from build123d import *

# Parameters (mm, degrees)
SKETCH_1_R          = 1.5
EXTRUDE_1_DEPTH     = 40
SKETCH_2_R          = 2.75
EXTRUDE_2_DEPTH     = 2.93
CUT_EXTRUDE_1_DEPTH = 1.3


with BuildPart() as part:
    # 草图1 → 凸台-拉伸1 (new body)
    with BuildSketch(Plane(origin=(0, 0, 0), x_dir=(1, 0, 0), z_dir=(0, 1, 0))):
        Circle(SKETCH_1_R)
    extrude(amount=EXTRUDE_1_DEPTH)

    # 草图2 → 凸台-拉伸2 (add)
    with BuildSketch(Plane(origin=(0, 40, 0), x_dir=(1, 0, 0), z_dir=(0, 1, 0))):
        Circle(SKETCH_2_R)
    extrude(amount=EXTRUDE_2_DEPTH)

    # 草图3 → 切除-拉伸1 (cut)
    with BuildSketch(Plane(origin=(0, 42.93, 0), x_dir=(1, 0, 0), z_dir=(0, 1, 0))):
        Polygon((1.024005842, -1.017224346), (1.392945046, 0.378202899), (0.368939204, 1.395427245), (-1.024005842, 1.017224346), (-1.392945046, -0.378202899), (-0.368939204, -1.395427245), align=None)
    extrude(amount=-CUT_EXTRUDE_1_DEPTH, mode=Mode.SUBTRACT)


solid = part.part
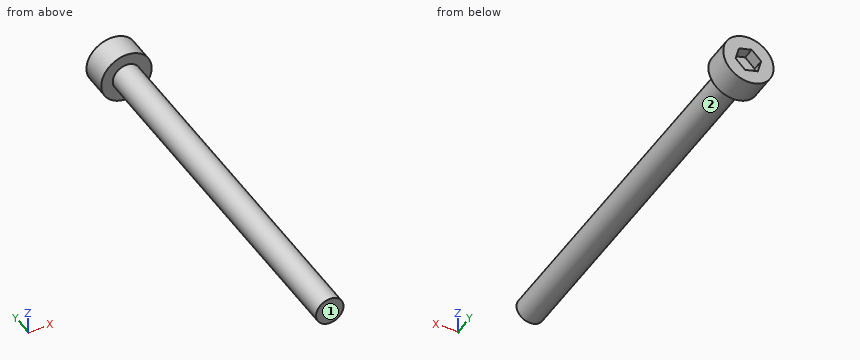
Here's how the part is built. I have some questions about the finished solid (model axes, mm). Face numbers are marked on the shaded views. A direction names the side the tool comes from. Round coordinates to 2 decimals unless told otherwise and drop trailing zeros. Write each loop counter-clockwise with the first axis right and the second up, starting at its lowest first coordinate (ties: lowest second). Pieces come first, ordered by that corner, then holes.
1. Suppose I cut it at A-A (x = 0). List the corners of the cut face in (y, z) for me, and give its area (3 significant figures).
2. Will these pins go through, and if not, where does the flat tip stop? pin 1 Ø1 at (y, z) = (32.5, 0) entering from +X; pin 2 Ø1 at (y, z) = (23.5, 1.5) entering from -X.
3. Suppose I cut it at D-D (z = -2.3). List the corners of the cut face in (x, y) for me.
4. Suppose I cut it at B-B (y = 16). List the corners of the cut face in (x, z) for me.
5. For the marked faces 1 and 2, which set-ups out of +Z, -Z, +X, -X, +Y, -Y let a thin tool reach every point of the face, with its end or its side?
6. Suppose I cut it at C-C (z = 0). List the corners of the cut face in (x, y) for me.
7. I need wall thicknesses on L1, parallel to X at y = 32.5, z = 1.1; L2, parallel to Y at x = 0.5, z = 0.7; L3, parallel to Y at x = -1.1, z = -2. Which ranges of each line are inside material? Lowest first, please.
Answer sheet:
1. outline: (0, -1.5) - (40, -1.5) - (40, -2.75) - (42.93, -2.75) - (42.93, -1.3) - (41.63, -1.3) - (41.63, 1.3) - (42.93, 1.3) - (42.93, 2.75) - (40, 2.75) - (40, 1.5) - (0, 1.5) - close
1. area: 133 mm2
2. pin 1: stops at x = 1.5
2. pin 2: stops at x = -1.12
3. outline: (-1.51, 40) - (1.51, 40) - (1.51, 42.93) - (-1.51, 42.93) - close
4. outline: circle Ø3 at (0, 0)
5. face 1: +Z, -Z, +X, -X, -Y
5. face 2: -Y
6. outline: (-2.75, 40) - (-1.5, 40) - (-1.5, 0) - (1.5, 0) - (1.5, 40) - (2.75, 40) - (2.75, 42.93) - (1.29, 42.93) - (1.29, 41.63) - (-1.29, 41.63) - (-1.29, 42.93) - (-2.75, 42.93) - close
7. L1: x = -1.02 to 1.02
7. L2: y = 0 to 41.63
7. L3: y = 40 to 42.93
